```python
from build123d import *

# Parameters (mm, degrees)
SKETCH1_R           = 2
BOSS_EXTRUDE1_DEPTH = 1


with BuildPart() as part:
    # Sketch1 → Boss-Extrude1 (new body)
    with BuildSketch(Plane(origin=(0, 0, 0), x_dir=(1, 0, 0), z_dir=(0, 1, 0))):
        with BuildLine():
            Line((-5.5, 0), (-54.5, 0))
            ThreePointArc((-54.5, 0), (-60, 5.5), (-54.5, 11))
            Line((-54.5, 11), (-5.5, 11))
            ThreePointArc((-5.5, 11), (0, 5.5), (-5.5, 0))
        make_face()
        with Locations((-52.5, 5)):
            Circle(SKETCH1_R, mode=Mode.SUBTRACT)
        with Locations((-37.5, 5)):
            Circle(SKETCH1_R, mode=Mode.SUBTRACT)
        with Locations((-22.5, 5)):
            Circle(SKETCH1_R, mode=Mode.SUBTRACT)
        with Locations((-7.5, 5)):
            Circle(SKETCH1_R, mode=Mode.SUBTRACT)
    extrude(amount=BOSS_EXTRUDE1_DEPTH)


solid = part.part
```
For this review, take the finished solid that the model builds, in its own axes (mm). Round coordinates to 2 decimals unless told otherwise and drop trailing zeros. Write each loop counter-clockwise with the first axis right and the second up, starting at its lowest first coordinate (ties: lowest second). Pieces come first, ordered by that corner, then holes. Notation, with made-up numbers: (51.5, 49) - (98.5, 49) arc R26 ccw to (98.5, 79) - close; hole circle Ø10 at (-6.75, -40). An arc over 180 degrees is marked (long way). Write each question's results on one line, items separated by ' | '.
Item 1: To check wall thickness, follow line 1 along Z through (x, y) = (-52.5, 0.4); line 2 along X through (y, z) = (0.5, -5.5); line 3 along X through (y, z) = (0.7, -5). State the ranges of each line that lie inside material, in increasing order. Write a range as from..to.
Calculated:
line 1: z = -11..-7, -3..0 | line 2: x = -60..-54.44, -50.56..-39.44, -35.56..-24.44, -20.56..-9.44, -5.56..0 | line 3: x = -59.98..-54.5, -50.5..-39.5, -35.5..-24.5, -20.5..-9.5, -5.5..-0.02
Item 2: For pin 1 (3 mm diameter, centred on x = -7.5, z = -5, fed in from +Y), flat-tipped, find the tip position at first contact; note if it passes through.
Calculated:
pin 1: passes through
Item 3: Take a section at C-C on z = -5. State the section outline as (x, y) points.
Calculated:
outline: (-59.98, 0) - (-54.5, 0) - (-54.5, 1) - (-59.98, 1) - close; (-50.5, 0) - (-39.5, 0) - (-39.5, 1) - (-50.5, 1) - close; (-35.5, 0) - (-24.5, 0) - (-24.5, 1) - (-35.5, 1) - close; (-20.5, 0) - (-9.5, 0) - (-9.5, 1) - (-20.5, 1) - close; (-5.5, 0) - (-0.02, 0) - (-0.02, 1) - (-5.5, 1) - close
Item 4: Draft analysis for pull direction X (two halves, no side actions). For faces 1 (the face through (-60, 0.5, -5.4)), 2 (the face through (-24.498, 0.493, -5.088)), 3 (the face through (-29.7, 0.5, 0)), state which applies: pulls with the +X half, pulls with the -X half, needs draft (parallel to the pull), parting line crosses it, or undercut.
Calculated:
face 1: pulls with the -X half | face 2: undercut | face 3: needs draft
Item 5: Take a section at B-B on y = 0.6. State the section outline as (x, z) points, then the cut area to 3 significant figures.
Calculated:
outline: (-54.5, -11) - (-5.5, -11) arc R5.5 ccw to (-5.5, 0) - (-54.5, 0) arc R5.5 ccw to start; hole circle Ø4 at (-52.5, -5); hole circle Ø4 at (-37.5, -5); hole circle Ø4 at (-22.5, -5); hole circle Ø4 at (-7.5, -5) | area: 584 mm^2
Item 6: Take a section at A-A on x = -7.5. State the section outline as (y, z) points, then the cut area to 3 significant figures.
Calculated:
outline: (0, -11) - (1, -11) - (1, -7) - (0, -7) - close; (0, -3) - (1, -3) - (1, 0) - (0, 0) - close | area: 7.00 mm^2
Item 7: Take a section at D-D on z = -2.25. State the section outline as (x, y) points, then the cut area to 3 significant figures.
Calculated:
outline: (-58.94, 0) - (-1.06, 0) - (-1.06, 1) - (-58.94, 1) - close | area: 57.9 mm^2
